Geometry check sheet. Reference: the model listing, model coordinates, mm. Face numbers are marked on the shaded views. Round coordinates to 2 decimals unless told otherwise and drop trailing zeros. Write each loop counter-clockwise with the first axis right and the second up, starting at its lowest first coordinate (ties: lowest second). Pieces come first, ordered by that corner, then holes. Notation, with made-up numbers: M 12.5,67.5 L 27.5,67.5 A29 ccw 27.5,101.5 Z; hole C 26,-18.5 d4. An arc over 180 degrees is marked long. One line per item, written item: value. Start each with the question number.
1. Section check A-A (y = 0). Record the boundary of the cut face in (x, z), and give its area (3 significant figures).
2. Section check C-C (z = 7). Record the boundary of the cut face in (x, y).
3. Section check D-D (z = 23.5). Record the boundary of the cut face in (x, y).
4. Scan lines: probe 1 along Y at (x, z) = (0, 5); probe 2 along X at (y, z) = (14.5, 6.5); probe 3 along X at (y, z) = (4, 2.75). Record each from-to range of solid material in increasing order. Write a range as [from, to].
5. Release check for a two-part mould opening along Y. For the marked faces 1, 2 and 3 record: pulls with the +Y half, pulls with the -Y half, needs draft (parallel to the pull), parting line crosses it, or undercut.
6. Depth check by flat-ended pin: P1, Ø1.5, axis at x = -2.5, z = 16, coming from the +Y side; P2, Ø1, axis at x = -4.5, z = 12, coming from the +Y side; P3, Ø1.5, axis at x = 26, y = 17.5, coming from the -Z side. Enter the tip coordinate at first touch or a pass-through.
from build123d import *

# Parameters (mm, degrees)
SKETCH_1_R               = 32.5
EXTRUDE_1_DEPTH          = 25.5
CUT_EXTRUDE_1_DEPTH      = 53.561868308
CUT_EXTRUDE_1_DEPTH_BACK = 53.561868308
SKETCH_2_R               = 25
FILLET_1_R               = 3
FILLET_2_R               = 3


with BuildPart() as part:
    # 草图1 → 凸台-拉伸1 (new body)
    with BuildSketch(Plane.XY):
        Circle(SKETCH_1_R)
    extrude(amount=EXTRUDE_1_DEPTH)

    # 草图2 → 切除-拉伸1 (cut, two sides: drawn at the far end of the back side and taken through both)
    with BuildSketch(Plane.XY.offset(25.5).offset(-CUT_EXTRUDE_1_DEPTH_BACK)):
        Circle(SKETCH_2_R)
    extrude(amount=CUT_EXTRUDE_1_DEPTH + CUT_EXTRUDE_1_DEPTH_BACK, mode=Mode.SUBTRACT)

    # 圆角1
    fillet_1_edges = [part.edges().sort_by_distance(p)[0] for p in [
        (-32.5, 0, 25.5),
    ]]
    fillet(fillet_1_edges, radius=FILLET_1_R)

    # 圆角2
    fillet_2_edges = [part.edges().sort_by_distance(p)[0] for p in [
        (-32.5, 0, 0),
    ]]
    fillet(fillet_2_edges, radius=FILLET_2_R)


solid = part.part
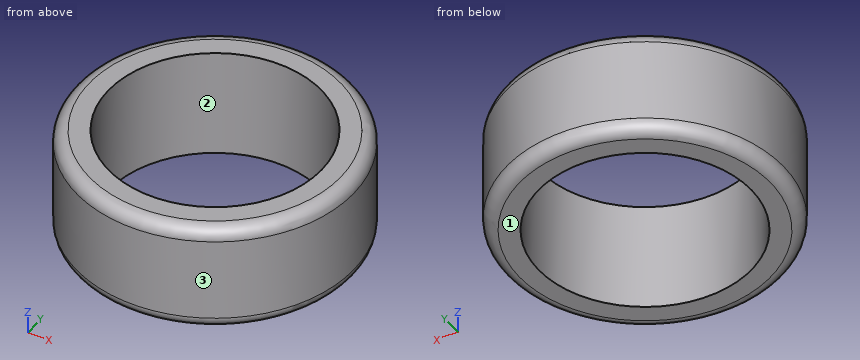
Result sheet:
1. outline: M -32.5,3 A3 ccw -29.5,0 L -25,0 L -25,25.5 L -29.5,25.5 A3 ccw -32.5,22.5 Z; M 25,0 L 29.5,0 A3 ccw 32.5,3 L 32.5,22.5 A3 ccw 29.5,25.5 L 25,25.5 Z
1. area: 375 mm2
2. outline: C 0,0 d65; hole C 0,0 d50
3. outline: C 0,0 d64.66; hole C 0,0 d50
4. probe 1: y = [-32.5, -25], [25, 32.5]
4. probe 2: x = [-29.09, -20.37], [20.37, 29.09]
4. probe 3: x = [-32.24, -24.68], [24.68, 32.24]
5. face 1: needs draft
5. face 2: undercut
5. face 3: parting line crosses it
6. P1: stops at y = 32.45
6. P2: stops at y = 32.25
6. P3: stops at z = 0.21
